The figure shows three views and two pictorial views of one solid part (mm, origin at its lowest corner). Answer the questions. A direction names the side the tool comes from. Coordinates: 2 decimals unless noted, no trailing zeros. Loops run counter-clockwise (first coordinate to the right, second up) from the corner with the lowest first, then second, coordinate; pieces in that order, holes last. Notation, with made-up numbers: (4, 50.25) - (61, 50.25) arc R12 cw to (61, 58.25) - close; hole circle Ø2 at (89.5, 42). An arc over 180 degrees is marked (long way). One line per question, with ' | ' between items.
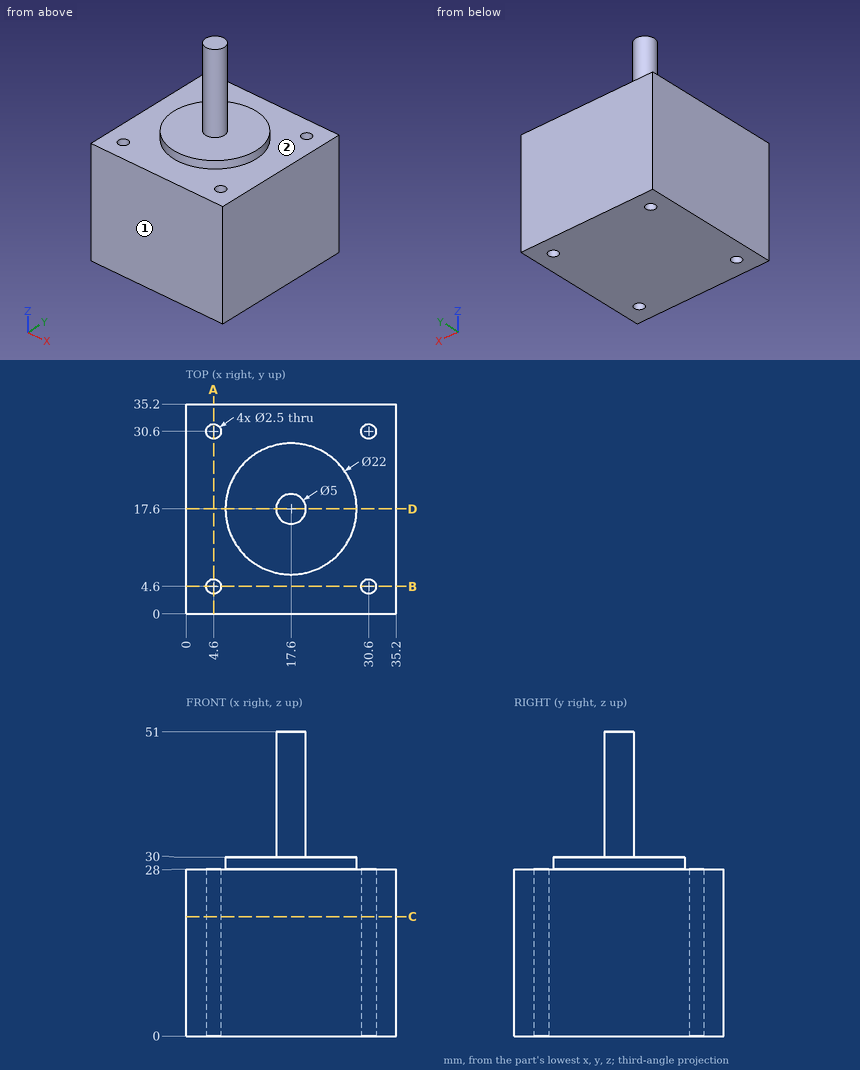
Item 1: Find the intervals of material crossed by line 1 (Y direction, x = 30.6, z = 21); line 2 (X direction, y = 3.5, z = 18); line 3 (X direction, y = 30, z = 7), in increasing order. Write a range as [from, to].
Taken from the geometry:
line 1: y = [0, 3.35], [5.85, 29.35], [31.85, 35.2] | line 2: x = [0, 4.01], [5.19, 30.01], [31.19, 35.2] | line 3: x = [0, 3.5], [5.7, 29.5], [31.7, 35.2]
Item 2: Each of these flat-tipped pins is pushed along its axis until it touches: pin 1 Ø1 at (x, y) = (30.5, 9) entering from +Z; pin 2 Ø2 at (x, y) = (30.6, 30.6) entering from +Z. Where does it stop, or does it pass through?
Taken from the geometry:
pin 1: stops at z = 28 | pin 2: passes through
Item 3: Find section D-D, the plane y = 17.6. Write down the section's boundary in (x, z), plus the area to 3 significant figures.
Taken from the geometry:
outline: (0, 0) - (35.2, 0) - (35.2, 28) - (28.6, 28) - (28.6, 30) - (20.1, 30) - (20.1, 51) - (15.1, 51) - (15.1, 30) - (6.6, 30) - (6.6, 28) - (0, 28) - close | area: 1,130 mm2
Item 4: Find section C-C, the plane z = 20. Write down the section's boundary in (x, y).
Taken from the geometry:
outline: (0, 0) - (35.2, 0) - (35.2, 35.2) - (0, 35.2) - close; hole circle Ø2.5 at (4.6, 4.6); hole circle Ø2.5 at (4.6, 30.6); hole circle Ø2.5 at (30.6, 4.6); hole circle Ø2.5 at (30.6, 30.6)
Item 5: Which of the six approach directions +Z, -Z, +X, -X, +Y, -Y give full straight-line access (tool end or side, diameter ignored) to the marked faces 1 and 2?
Taken from the geometry:
face 1: +Z, -Z, +X, -X, -Y | face 2: +Z
Item 6: Find section A-A, the plane x = 4.6. Write down the section's boundary in (y, z), plus the area to 3 significant figures.
Taken from the geometry:
outline: (0, 0) - (3.35, 0) - (3.35, 28) - (0, 28) - close; (5.85, 0) - (29.35, 0) - (29.35, 28) - (5.85, 28) - close; (31.85, 0) - (35.2, 0) - (35.2, 28) - (31.85, 28) - close | area: 846 mm2
